For this review, take the finished solid that the model builds, in its own axes (mm). Give positions to 0.01 mm unless a question says otherwise; leave off trailing zeros. Write each loop counter-clockwise with the first axis right and the second up, starting at its lowest first coordinate (ties: lowest second). Pieces come first, ordered by that corner, then holes.
1) We need section B-B on z = 0. Give the boundary of the cut face in (x, y).
2) Wall thickness on line 1 along X through (y, z) = (1.75, -8); line 2 along Y through (x, z) = (-8.5, -17.5); line 3 along X through (y, z) = (20.75, 44.5): over which ranges is each line inside the solid? List them lowest first.
3) We need section A-A on x = 0. Give the number of separate pieces and of enclosed holes in the cut face, and give its area (3 significant figures).
4) We need section D-D on z = -18. Give the boundary of the cut face in (x, y), and give its area (3 significant figures).
5) We need section C-C on x = -49.5. Give the boundary of the cut face in (y, z), and give its area (3 significant figures).
6) For P1, Ø0.8, axis at x = 58, y = 26, coming from the +Z side; P2, Ø3, axis at y = 12, z = 38.5, coming from the +X side; P3, Ø2.5, axis at x = -43.5, y = 2, coming from the -Z side; P4, Ø7.5, axis at x = -29.5, z = 51.5, coming from the -Y side, all flat-tipped, find the tip position at first contact; note any pin that passes through.
from build123d import *
from build123d.topology import SkipClean

# Parameters (mm, degrees)
SKETCH_1_R          = 1.5
SKETCH_1_R_2        = 5
EXTRUDE_1_DEPTH     = 3
SKETCH_2_R          = 57.5
SKETCH_2_R_2        = 55
EXTRUDE_2_DEPTH     = 25
EXTRUDE_START       = -3
SKETCH_3_R          = 1.5
EXTRUDE_3_DEPTH     = 3
CUT_EXTRUDE_START   = -30
SKETCH_4_R          = 69.475087651
SKETCH_4_R_2        = 57.5
CUT_EXTRUDE_1_DEPTH = 30


with BuildPart() as part:
    # Sketch 1 → Extrude 1 (new body)
    with BuildSketch(Plane(origin=(0, 0, 0), x_dir=(1, 0, 0), z_dir=(0, 1, 0))):
        with BuildLine():
            Line((57.421685799, 3), (60, 3))
            ThreePointArc((60, 3), (63, 0), (60, -3))
            Line((60, -3), (57.421685799, -3))
            ThreePointArc((57.421685799, -3), (28.75, -49.796460718), (-26.112766688, -51.22863863))
            Line((-26.112766688, -51.22863863), (-27.401923789, -53.461524227))
            ThreePointArc((-27.401923789, -53.461524227), (-31.5, -54.559600438), (-32.598076211, -50.461524227))
            Line((-32.598076211, -50.461524227), (-31.308919111, -48.22863863))
            ThreePointArc((-31.308919111, -48.22863863), (-57.5, 0), (-31.308919111, 48.22863863))
            Line((-31.308919111, 48.22863863), (-32.598076211, 50.461524227))
            ThreePointArc((-32.598076211, 50.461524227), (-31.5, 54.559600438), (-27.401923789, 53.461524227))
            Line((-27.401923789, 53.461524227), (-26.112766688, 51.22863863))
            ThreePointArc((-26.112766688, 51.22863863), (28.75, 49.796460718), (57.421685799, 3))
        make_face()
        with Locations(Location((0, 8, 0), (0, 0, 270))):
            Circle(SKETCH_1_R, mode=Mode.SUBTRACT)
        with Locations(Location((8, 0, 0), (0, 0, 270))):
            Circle(SKETCH_1_R, mode=Mode.SUBTRACT)
        with Locations(Location((0, -8, 0), (0, 0, 270))):
            Circle(SKETCH_1_R, mode=Mode.SUBTRACT)
        with Locations(Location((-8, 0, 0), (0, 0, 270))):
            Circle(SKETCH_1_R, mode=Mode.SUBTRACT)
        with Locations(Location((0, 0, 0), (0, 0, 270))):
            Circle(SKETCH_1_R_2, mode=Mode.SUBTRACT)
        with Locations(Location((60, 0, 0), (0, 0, 270))):
            Circle(SKETCH_1_R, mode=Mode.SUBTRACT)
        with Locations(Location((-30, -51.961524227, 0), (0, 0, 270))):
            Circle(SKETCH_1_R, mode=Mode.SUBTRACT)
        with Locations(Location((-30, 51.961524227, 0), (0, 0, 270))):
            Circle(SKETCH_1_R, mode=Mode.SUBTRACT)
        with BuildLine():
            Line((10.583005244, 3), (29.849623113, 3))
            ThreePointArc((29.849623113, 3), (25.980762114, 15), (17.522887768, 24.350531909))
            Line((17.522887768, 24.350531909), (7.889578833, 7.66515139))
            ThreePointArc((7.889578833, 7.66515139), (9.526279442, 5.5), (10.583005244, 3))
        make_face(mode=Mode.SUBTRACT)
        with BuildLine():
            Line((10.583005244, -3), (29.849623113, -3))
            ThreePointArc((29.849623113, -3), (25.980762114, -15), (17.522887768, -24.350531909))
            Line((17.522887768, -24.350531909), (7.889578833, -7.66515139))
            ThreePointArc((7.889578833, -7.66515139), (9.526279442, -5.5), (10.583005244, -3))
        make_face(mode=Mode.SUBTRACT)
        with BuildLine():
            Line((2.693426411, -10.66515139), (12.326735345, -27.350531909))
            ThreePointArc((12.326735345, -27.350531909), (0, -30), (-12.326735345, -27.350531909))
            Line((-12.326735345, -27.350531909), (-2.693426411, -10.66515139))
            ThreePointArc((-2.693426411, -10.66515139), (0, -11), (2.693426411, -10.66515139))
        make_face(mode=Mode.SUBTRACT)
        with BuildLine():
            Line((-14.837519563, 31.699337741), (-24.860984224, 49.060487802))
            ThreePointArc((-24.860984224, 49.060487802), (0, 55), (24.860984224, 49.060487802))
            Line((24.860984224, 49.060487802), (14.837519563, 31.699337741))
            ThreePointArc((14.837519563, 31.699337741), (0, 35), (-14.837519563, 31.699337741))
        make_face(mode=Mode.SUBTRACT)
        with BuildLine():
            Line((-7.889578833, -7.66515139), (-17.522887768, -24.350531909))
            ThreePointArc((-17.522887768, -24.350531909), (-25.980762114, -15), (-29.849623113, -3))
            Line((-29.849623113, -3), (-10.583005244, -3))
            ThreePointArc((-10.583005244, -3), (-9.526279442, -5.5), (-7.889578833, -7.66515139))
        make_face(mode=Mode.SUBTRACT)
        with BuildLine():
            Line((-10.583005244, 3), (-29.849623113, 3))
            ThreePointArc((-29.849623113, 3), (-25.980762114, 15), (-17.522887768, 24.350531909))
            Line((-17.522887768, 24.350531909), (-7.889578833, 7.66515139))
            ThreePointArc((-7.889578833, 7.66515139), (-9.526279442, 5.5), (-10.583005244, 3))
        make_face(mode=Mode.SUBTRACT)
        with BuildLine():
            Line((20.033671986, 28.699337741), (30.057136647, 46.060487802))
            ThreePointArc((30.057136647, 46.060487802), (47.631397208, 27.5), (54.918120871, 3))
            Line((54.918120871, 3), (34.871191548, 3))
            ThreePointArc((34.871191548, 3), (30.310889132, 17.5), (20.033671986, 28.699337741))
        make_face(mode=Mode.SUBTRACT)
        with BuildLine():
            Line((-20.033671986, 28.699337741), (-30.057136647, 46.060487802))
            ThreePointArc((-30.057136647, 46.060487802), (-47.631397208, 27.5), (-54.918120871, 3))
            Line((-54.918120871, 3), (-34.871191548, 3))
            ThreePointArc((-34.871191548, 3), (-30.310889132, 17.5), (-20.033671986, 28.699337741))
        make_face(mode=Mode.SUBTRACT)
        with BuildLine():
            Line((-2.693426411, 10.66515139), (-12.326735345, 27.350531909))
            ThreePointArc((-12.326735345, 27.350531909), (0, 30), (12.326735345, 27.350531909))
            Line((12.326735345, 27.350531909), (2.693426411, 10.66515139))
            ThreePointArc((2.693426411, 10.66515139), (0, 11), (-2.693426411, 10.66515139))
        make_face(mode=Mode.SUBTRACT)
        with BuildLine():
            Line((-34.871191548, -3), (-54.918120871, -3))
            ThreePointArc((-54.918120871, -3), (-47.631397208, -27.5), (-30.057136647, -46.060487802))
            Line((-30.057136647, -46.060487802), (-20.033671986, -28.699337741))
            ThreePointArc((-20.033671986, -28.699337741), (-30.310889132, -17.5), (-34.871191548, -3))
        make_face(mode=Mode.SUBTRACT)
        with BuildLine():
            Line((34.871191548, -3), (54.918120871, -3))
            ThreePointArc((54.918120871, -3), (47.631397208, -27.5), (30.057136647, -46.060487802))
            Line((30.057136647, -46.060487802), (20.033671986, -28.699337741))
            ThreePointArc((20.033671986, -28.699337741), (30.310889132, -17.5), (34.871191548, -3))
        make_face(mode=Mode.SUBTRACT)
        with BuildLine():
            Line((14.837519563, -31.699337741), (24.860984224, -49.060487802))
            ThreePointArc((24.860984224, -49.060487802), (0, -55), (-24.860984224, -49.060487802))
            Line((-24.860984224, -49.060487802), (-14.837519563, -31.699337741))
            ThreePointArc((-14.837519563, -31.699337741), (0, -35), (14.837519563, -31.699337741))
        make_face(mode=Mode.SUBTRACT)
    extrude(amount=EXTRUDE_1_DEPTH)

    # Sketch 2 → Extrude 2 (add)
    with SkipClean():  # the faces are left unmerged after this step: merging them gives an invalid solid
        with BuildSketch(Plane(origin=(0, 3, 0), x_dir=(1, 0, 0), z_dir=(0, 1, 0))):
            with Locations(Location((0, 0, 0), (0, 0, 117.009297093))):
                Circle(SKETCH_2_R)
            with Locations(Location((0, 0, 0), (0, 0, 63.126776114))):
                Circle(SKETCH_2_R_2, mode=Mode.SUBTRACT)
        extrude(amount=EXTRUDE_2_DEPTH)

    # Sketch 3 → Extrude 3 (add)
    # profile 1 of 3: a face of its own
    with SkipClean():  # the faces are left unmerged after this step: merging them gives an invalid solid
        with BuildSketch(Plane(origin=(0, 28, 0), x_dir=(1, 0, 0), z_dir=(0, 1, 0)).offset(EXTRUDE_START)):
            with BuildLine():
                Line((-32.598076211, 50.461524227), (-31.308919111, 48.22863863))
                ThreePointArc((-31.308919111, 48.22863863), (-28.75, 49.796460718), (-26.112766688, 51.22863863))
                Line((-26.112766688, 51.22863863), (-27.401923789, 53.461524227))
                ThreePointArc((-27.401923789, 53.461524227), (-31.5, 54.559600438), (-32.598076211, 50.461524227))
            make_face()
            with Locations(Location((-30, 51.961524227, 0), (0, 0, 270))):
                Circle(SKETCH_3_R, mode=Mode.SUBTRACT)
        # profile 2 of 3: a face of its own
        with BuildSketch(Plane(origin=(0, 28, 0), x_dir=(1, 0, 0), z_dir=(0, 1, 0)).offset(EXTRUDE_START)):
            with BuildLine():
                Line((60, 3), (57.421685799, 3))
                ThreePointArc((57.421685799, 3), (57.5, 0), (57.421685799, -3))
                Line((57.421685799, -3), (60, -3))
                ThreePointArc((60, -3), (63, 0), (60, 3))
            make_face()
            with Locations(Location((60, 0, 0), (0, 0, 270))):
                Circle(SKETCH_3_R, mode=Mode.SUBTRACT)
        # profile 3 of 3: a face of its own
        with BuildSketch(Plane(origin=(0, 28, 0), x_dir=(1, 0, 0), z_dir=(0, 1, 0)).offset(EXTRUDE_START)):
            with BuildLine():
                Line((-27.401923789, -53.461524227), (-26.112766688, -51.22863863))
                ThreePointArc((-26.112766688, -51.22863863), (-28.75, -49.796460718), (-31.308919111, -48.22863863))
                Line((-31.308919111, -48.22863863), (-32.598076211, -50.461524227))
                ThreePointArc((-32.598076211, -50.461524227), (-31.5, -54.559600438), (-27.401923789, -53.461524227))
            make_face()
            with Locations(Location((-30, -51.961524227, 0), (0, 0, 270))):
                Circle(SKETCH_3_R, mode=Mode.SUBTRACT)
        extrude(amount=EXTRUDE_3_DEPTH)

    # Sketch 4 → Cut-Extrude 1 (cut)
    with SkipClean():  # the faces are left unmerged after this step: merging them gives an invalid solid
        with BuildSketch(Plane(origin=(0, 3, 0), x_dir=(1, 0, 0), z_dir=(0, 1, 0)).offset(CUT_EXTRUDE_START)):
            Circle(SKETCH_4_R)
            with Locations(Location((0, 0, 0), (0, 0, 117.009297093))):
                Circle(SKETCH_4_R_2, mode=Mode.SUBTRACT)
        extrude(amount=CUT_EXTRUDE_1_DEPTH, mode=Mode.SUBTRACT)
    add(part.part.scale(1), mode=Mode.REPLACE)  # the faces are merged on a copy


solid = part.part
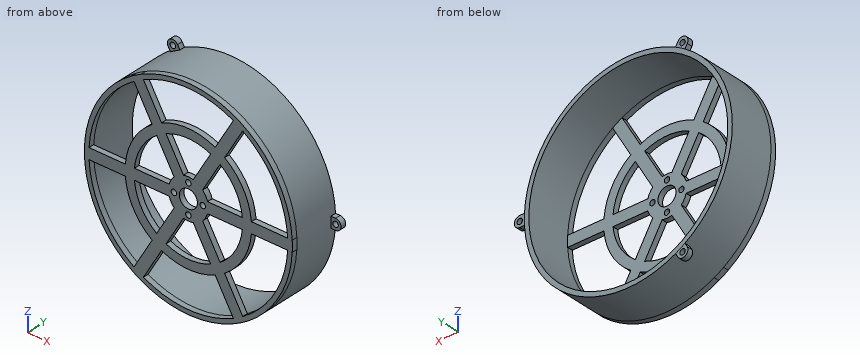
Results list:
1. outline: (-57.5, 0) - (-9.5, 0) - (-9.5, 3) - (-55, 3) - (-55, 28) - (-57.5, 28) - close; (-6.5, 0) - (-5, 0) - (-5, 3) - (-6.5, 3) - close; (5, 0) - (6.5, 0) - (6.5, 3) - (5, 3) - close; (9.5, 0) - (57.5, 0) - (57.5, 25) - (58.5, 25) - (58.5, 28) - (55, 28) - (55, 3) - (9.5, 3) - close; (61.5, 25) - (63, 25) - (63, 28) - (61.5, 28) - close
2. line 1: x = -56.94 to -54.42, -34.07 to -28.91, -8.08 to -1.5, 1.5 to 8.08, 28.91 to 34.07, 54.42 to 56.94
2. line 2: y = 0 to 3
2. line 3: x = -36.41 to -32.32, 32.32 to 36.41
3. separate pieces: 8
3. enclosed holes: 0
3. area: 188 mm2
4. outline: (-54.61, 0) - (-51.97, 0) - (-51.97, 28) - (-54.61, 28) - close; (-30.02, 0) - (-24, 0) - (-24, 3) - (-30.02, 3) - close; (-13.86, 0) - (-6.93, 0) - (-6.93, 3) - (-13.86, 3) - close; (6.93, 0) - (13.86, 0) - (13.86, 3) - (6.93, 3) - close; (24, 0) - (30.02, 0) - (30.02, 3) - (24, 3) - close; (51.97, 0) - (54.61, 0) - (54.61, 28) - (51.97, 28) - close
4. area: 225 mm2
5. outline: (0, -29.26) - (28, -29.26) - (28, -23.97) - (0, -23.97) - close; (0, -3) - (3, -3) - (3, 3) - (0, 3) - close; (0, 23.97) - (28, 23.97) - (28, 29.26) - (0, 29.26) - close
5. area: 314 mm2
6. P1: stops at z = 3
6. P2: stops at x = 44.01
6. P3: stops at z = -39
6. P4: stops at y = 0
